Autodesk Inventor part; units mm, degrees
ref_plane "YZ Plane" through (0, 0, 0) normal (1, 0, 0) x (0, 1, 0)
ref_plane "XZ Plane" through (0, 0, 0) normal (0, 1, 0) x (-1, 0, 0)
ref_plane "XY Plane" through (0, 0, 0) normal (0, 0, 1) x (1, 0, 0)
sketch "Skizze2" plane through (0, 0, 0) normal (0, 0, 1) x (1, 0, 0)
  line L0 (-50, 75) -> (50, 75)
  line L1 (50, 75) -> (50, -75)
  line L2 (50, -75) -> (-50, -75)
  line L3 (-50, -75) -> (-50, 75)
  line L4 (-28.5786, 75) -> (-170, 216.4214)
  line L5 (-170, 216.4214) -> (-192, 194.4214)
  line L6 (-192, 194.4214) -> (-50, 52.4214)
  circle A0 centre (-181, 205.4214) radius 15.5563
  line L7 (28.5786, 75) -> (170, 216.4214)
  line L8 (170, 216.4214) -> (192, 194.4214)
  line L9 (192, 194.4214) -> (50, 52.4214)
  line L10 (50, -53) -> (192, -195)
  line L11 (192, -195) -> (170, -217)
  line L12 (170, -217) -> (28, -75)
  line L13 (-50, -53) -> (-192, -195)
  line L14 (-192, -195) -> (-170, -217)
  line L15 (-170, -217) -> (-28, -75)
  circle A1 centre (181, -206) radius 15.5563
  circle A2 centre (181, 205.4214) radius 15.5563
  circle A3 centre (-181, -206) radius 15.5563
  point P0 (0, 0)
  point P1 (50, 0)
  point P2 (0, 75)
  dimension "d0" = 150
  dimension "d1" = 100
  dimension "d2" = 135
  dimension "d4" = 22
  dimension "d6" = 200
  dimension "d7" = 120
  dimension "d8" = 31.1127
  dimension "d9" = 135
  dimension "d10" = 0
  dimension "d12" = 22
  dimension "d14" = 200
  dimension "d15" = 120
  dimension "d16" = 135
  dimension "d17" = 22
  dimension "d20" = 120
  dimension "d21" = 120
  dimension "d22" = 22
  dimension "d23" = 120
  dimension "d24" = 135
  dimension "d25" = 120
extrude "Extrusion1" add sketch "Skizze2" along normal blind 40
sketch "Skizze3" plane through (0, 0, 40) normal (0, 0, 1) x (1, 0, 0)
  arc A0 (-170, 216.4214) -> (-192, 194.4214) centre (-181, 205.4214) ccw
  circle A1 centre (-181, 205.4214) radius 11
  arc A2 (192, 194.4214) -> (170, 216.4214) centre (181, 205.4214) ccw
  circle A3 centre (181, 205.4214) radius 11
  arc A4 (170, -217) -> (192, -195) centre (181, -206) ccw
  circle A5 centre (181, -206) radius 11
  arc A6 (-192, -195) -> (-170, -217) centre (-181, -206) ccw
  circle A7 centre (-181, -206) radius 11
  point P0 (0, 0)
  dimension "d28" = 22
  dimension "d29" = 22
  dimension "d30" = 22
  dimension "d31" = 22
extrude "Extrusion2" cut sketch "Skizze3" against normal blind 20
sketch "Skizze4" plane through (0, 0, 40) normal (0, 0, 1) x (1, 0, 0)
  point P0 (0, 0)
properties part number "DrohneSkizze"
Read the model definition and answer for the solid it produces. Units are mm, in the model's axes. A direction names the side the tool comes from. Round coordinates to 2 decimals unless told otherwise and drop trailing zeros. Write each loop counter-clockwise with the first axis right and the second up, starting at its lowest first coordinate (ties: lowest second). Pieces come first, ordered by that corner, then holes.
1. The part is cut by section A-A, the plane y = -206. Determine the outline of the cut face in (x, z).
2. The part is cut by section B-B, the plane x = 181. Determine the outline of the cut face in (y, z), then the cut area to 3 significant figures.
3. The part is cut by section D-D, the plane z = 5. Determine the outline of the cut face in (x, y), then the cut area to 3 significant figures.
4. Which of the six approach directions +Z, -Z, +X, -X, +Y, -Y give full straight-line access (tool end or side, diameter ignored) to faces 4 (the face through (120, -123, 20)), 5 (the face through (-100, -147, 20)), 6 (the face through (-189.73, 198.73, 30.14)), 7 (the face through (-120, -123, 20))?
5. Given pin 1 Ø1.5 at (x, z) = (-68.5, 13.5) entering from -Y; pin 2 Ø3 at (y, z) = (-81.5, 9) entering from -X; pin 3 Ø3 at (x, z) = (69.5, 25.5) entering from +Y; pin 4 Ø24 at (x, y) = (181, -202.5) entering from +Z, each flat-ended and moving along its own axis, determine where each tip first touches the part or whether it passes through.
6. Determine the mould class of faces 1 (the face through (0, -75, 20)), 2 (the face through (-1, 1, 40)), 3 (the face through (121.994, 124.415, 19.72)) for opening direction X: pulls with the +X half, pulls with the -X half, needs draft (parallel to the pull), parting line crosses it, or undercut.
7. Straight lines are drawn through the part: L1, parallel to Y at x = -181, z = 25.75; L2, parallel to X at y = 30, z = 6; L3, parallel to Y at x = -7.5, z = 17.5. For each, find the intervals that lie inside material, in ascending order.
8. The part is cut by section C-C, the plane z = 26. Determine the outline of the cut face in (x, y), then the cut area to 3 significant figures.
Values:
1. outline: (-196.56, 0) - (-159, 0) - (-159, 40) - (-170, 40) - (-170, 20) - (-192, 20) - (-192, 40) - (-196.56, 40) - close; (159, 0) - (196.56, 0) - (196.56, 40) - (192, 40) - (192, 20) - (170, 20) - (170, 40) - (159, 40) - close
2. outline: (-221.56, 0) - (-184, 0) - (-184, 40) - (-195, 40) - (-195, 20) - (-217, 20) - (-217, 40) - (-221.56, 40) - close; (183.42, 0) - (220.98, 0) - (220.98, 40) - (216.42, 40) - (216.42, 20) - (194.42, 20) - (194.42, 40) - (183.42, 40) - close
2. area: 2,120 mm2
3. outline: (-192, -195) arc R15.56 ccw to (-170, -217) - (-28, -75) - (28, -75) - (170, -217) arc R15.56 ccw to (192, -195) - (50, -53) - (50, 52.42) - (192, 194.42) arc R15.56 ccw to (170, 216.42) - (28.58, 75) - (-28.58, 75) - (-170, 216.42) arc R15.56 ccw to (-192, 194.42) - (-50, 52.42) - (-50, -53) - close
3. area: 40,500 mm2
4. face 4: +Z, -Z, +X
4. face 5: +Z, -Z, -Y
4. face 6: +Z
4. face 7: +Z, -Z, -X
5. pin 1: stops at y = -116.25
5. pin 2: stops at x = -80
5. pin 3: stops at y = 117.42
5. pin 4: stops at z = 40
6. face 1: undercut
6. face 2: needs draft
6. face 3: pulls with the +X half
7. L1: y = -221.56 to -217, -195 to -184, 183.42 to 194.42, 216.42 to 220.98
7. L2: x = -50 to 50
7. L3: y = -75 to 75
8. outline: (-192, -195) arc R15.56 ccw to (-170, -217) - (-28, -75) - (28, -75) - (170, -217) arc R15.56 ccw to (192, -195) - (50, -53) - (50, 52.42) - (192, 194.42) arc R15.56 ccw to (170, 216.42) - (28.58, 75) - (-28.58, 75) - (-170, 216.42) arc R15.56 ccw to (-192, 194.42) - (-50, 52.42) - (-50, -53) - close; hole circle Ø22 at (-181, -206); hole circle Ø22 at (-181, 205.42); hole circle Ø22 at (181, -206); hole circle Ø22 at (181, 205.42)
8. area: 39,000 mm2
